Here's the drawing with two shaded views (mm, measured from the low corner). I have some questions. A direction names the side the tool comes from. Give positions to 0.01 mm unless a question says otherwise; leave off trailing zeros. Loops run counter-clockwise (first coordinate to the right, second up) from the corner with the lowest first, then second, coordinate; pieces in that order, holes last. Notation, with made-up numbers: (-23.75, 22) -> (14.25, 22) arc R21 ccw to (14.25, 31) -> close; hole circle Ø4 at (48.5, 57). An arc over 180 degrees is marked (long way). Put each result on its own line as item: value.
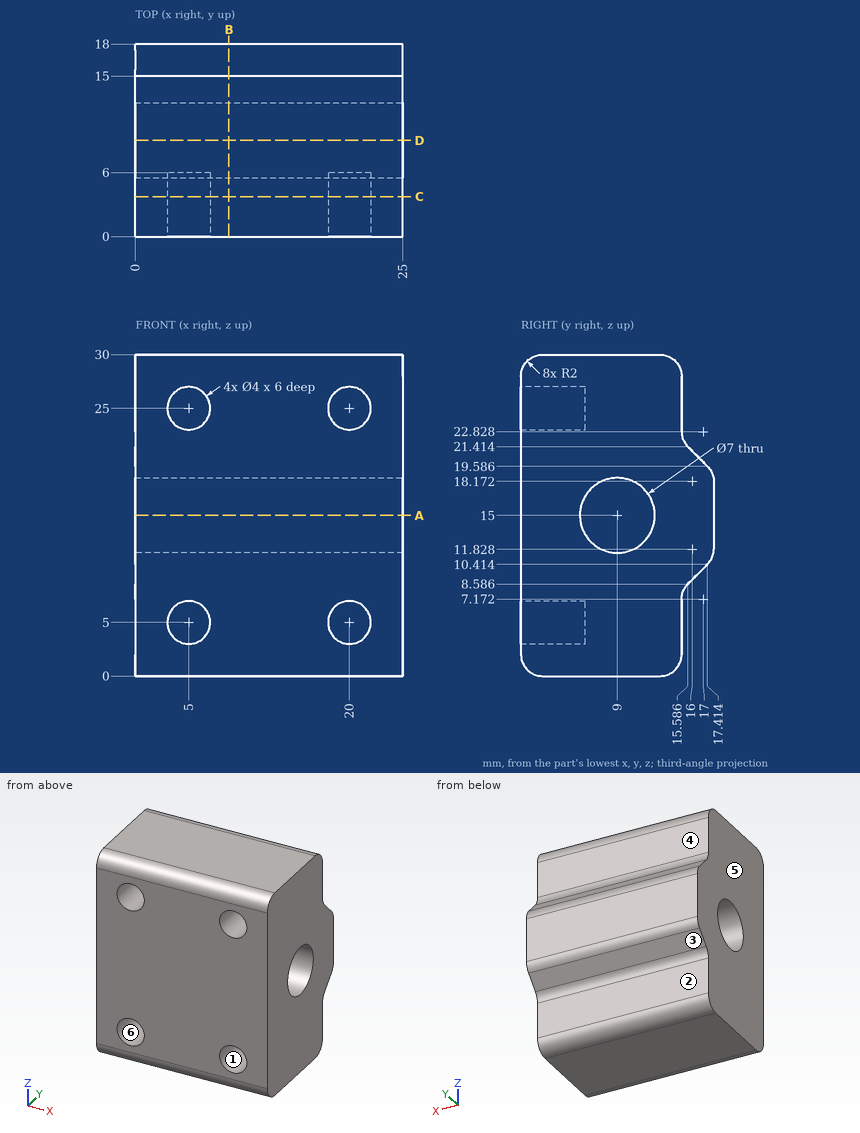
1. If we section it at D-D (y = 9): List the corners of the cut face in (x, z) for me, then the cut area to 3 significant figures.
Recorded:
outline: (0, 0) -> (25, 0) -> (25, 11.5) -> (0, 11.5) -> close; (0, 18.5) -> (25, 18.5) -> (25, 30) -> (0, 30) -> close
area: 575 mm^2
2. I need wall thicknesses on line 1 (X direction, y = 1.65, z = 5); line 2 (Z direction, x = 21.5, y = 4) (1 decimal); line 3 (Y direction, x = 14.75, z = 15). Which ranges of each line are inside material? Lowest first, please.
Recorded:
line 1: x = 0 to 3, 7 to 18, 22 to 25
line 2: z = 0 to 3.7, 6.3 to 23.7, 26.3 to 30
line 3: y = 0 to 5.5, 12.5 to 18
3. If we section it at B-B (x = 8.75): List the corners of the cut face in (y, z) for me (1 decimal), then the cut area to 3 significant figures.
Recorded:
outline: (0, 2) arc R2 ccw to (2, 0) -> (13, 0) arc R2 ccw to (15, 2) -> (15, 7.2) arc R2 cw to (15.6, 8.6) -> (17.4, 10.4) arc R2 ccw to (18, 11.8) -> (18, 18.2) arc R2 ccw to (17.4, 19.6) -> (15.6, 21.4) arc R2 cw to (15, 22.8) -> (15, 28) arc R2 ccw to (13, 30) -> (2, 30) arc R2 ccw to (0, 28) -> close; hole circle Ø7 at (9, 15)
area: 441 mm^2
4. If we section it at A-A (z = 15): List the corners of the cut face in (x, y) for me.
Recorded:
outline: (0, 0) -> (25, 0) -> (25, 5.5) -> (0, 5.5) -> close; (0, 12.5) -> (25, 12.5) -> (25, 18) -> (0, 18) -> close
5. I'm going to push flat-ended pins straight in: pin 1 (2.5 mm diameter, centred on x = 17.5, z = 26.5, fed in from +Y); pin 2 (2.5 mm diameter, centred on x = 20, z = 5, fed in from -Y); pin 3 (6.5 mm diameter, centred on y = 9, z = 15, fed in from +X). Where does each tip first touch, or does it pass through?
Recorded:
pin 1: stops at y = 15
pin 2: stops at y = 6
pin 3: passes through
6. For the marked faces 4, 5 and 6, which set-ups out of +Z, -Z, +X, -X, +Y, -Y let a thin tool reach every point of the face, with its end or its side?
Recorded:
face 4: +Z, +X, -X, +Y
face 5: +Z, -Z, -X, +Y, -Y
face 6: -Y
7. Thinking about a two-plate mould opening in Z: for the marked faces 1, 2 and 3, which applies, pulls with the +Z half, pulls with the -Z half, needs draft (parallel to the pull), parting line crosses it, or undercut?
Recorded:
face 1: undercut
face 2: needs draft
face 3: pulls with the -Z half
8. If we section it at C-C (y = 3.75): List the corners of the cut face in (x, z) for me, then the cut area to 3 significant figures.
Recorded:
outline: (0, 0) -> (25, 0) -> (25, 30) -> (0, 30) -> close; hole circle Ø4 at (5, 5); hole circle Ø4 at (5, 25); hole circle Ø4 at (20, 5); hole circle Ø4 at (20, 25)
area: 700 mm^2
